Part print with two shaded views. Sizes in mm from the minimum x, y, z corner. Round coordinates to 2 decimals unless told otherwise and drop trailing zeros. Write each loop counter-clockwise with the first axis right and the second up, starting at its lowest first coordinate (ties: lowest second). Pieces come first, ordered by that corner, then holes. Notation, with made-up numbers: (1, -11) - (46, -11) arc R13 ccw to (46, 14) - close; hole circle Ø6 at (-32.75, 89.5). An arc over 180 degrees is marked (long way). Answer as a JSON object with one key per item and string values. Group by question number.
Item 1: Probe line 1 (Y direction, x = 35, z = 7.5); line 2 (X direction, y = 156.5, z = 12.5); line 3 (Y direction, x = 37, z = 7.25). List the from-to ranges inside material, lowest first. Write a range as from..to.
Item 2: Slice it at C-C, the plane z = 12.5. List the corners of the cut face in (x, y), then the cut area to 3 significant figures.
Item 3: Slice it at A-A, the plane x = 135. List the corners of the cut face in (y, z), then the cut area to 3 significant figures.
Item 4: Flat gauge pin, fed straight in: pin 1 (20.5 mm diameter, centred on x = 35, y = 55, fed in from +Z). Where does the tip first touch, or does it go through?
Item 5: Slice it at B-B, the plane y = 55. List the corners of the cut face in (x, z), then the cut area to 3 significant figures.
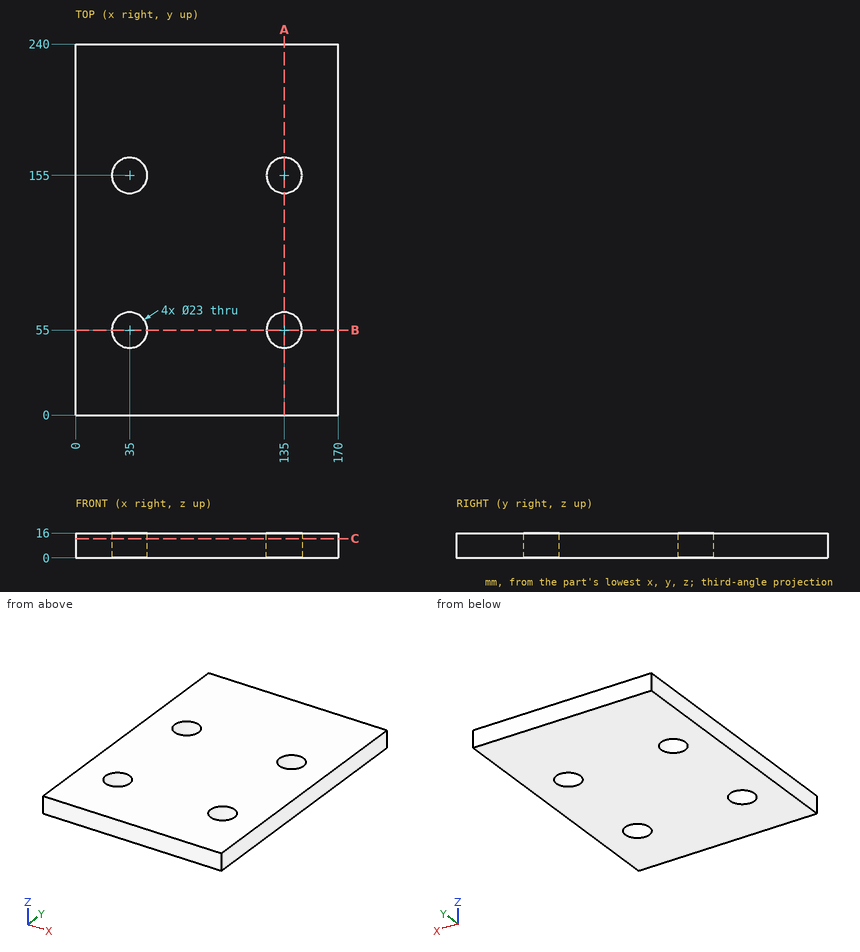
Geometry says:
{
 "1": {"line 1": "y = 0..43.5, 66.5..143.5, 166.5..240", "line 2": "x = 0..23.6, 46.4..123.6, 146.4..170", "line 3": "y = 0..43.68, 66.32..143.68, 166.32..240"},
 "2": {"outline": "(0, 0) - (170, 0) - (170, 240) - (0, 240) - close; hole circle Ø23 at (35, 55); hole circle Ø23 at (35, 155); hole circle Ø23 at (135, 55); hole circle Ø23 at (135, 155)", "area": "39,100 mm^2"},
 "3": {"outline": "(0, 0) - (43.5, 0) - (43.5, 16) - (0, 16) - close; (66.5, 0) - (143.5, 0) - (143.5, 16) - (66.5, 16) - close; (166.5, 0) - (240, 0) - (240, 16) - (166.5, 16) - close", "area": "3,100 mm^2"},
 "4": {"pin 1": "passes through"},
 "5": {"outline": "(0, 0) - (23.5, 0) - (23.5, 16) - (0, 16) - close; (46.5, 0) - (123.5, 0) - (123.5, 16) - (46.5, 16) - close; (146.5, 0) - (170, 0) - (170, 16) - (146.5, 16) - close", "area": "1,980 mm^2"}
}
